```python
from build123d import *

# Parameters (mm, degrees)
F2_R      = 4
F2_R_2    = 3.4
F5_DEPTH  = 14
F7_R      = 15
F3_R      = 4
F4_R      = 3.2
F8_R      = 14.2
F6_R      = 15
F6_R_2    = 14.4
F11_DEPTH = 44
F14_DEPTH = 2.4
F15_R     = 15
F16_DEPTH = 0.6


with BuildPart() as f5:
    # F2 (on Top) → F5 (new body)
    with BuildSketch(Plane.XY):
        Circle(F2_R)
        Circle(F2_R_2, mode=Mode.SUBTRACT)
    extrude(amount=F5_DEPTH)

    # F7 (on offset) → F9 section 0
    with BuildSketch(Plane.XY.offset(-10)):
        Circle(F7_R)
    # F3 (on Top) → F9 section 1
    with BuildSketch(Plane.XY):
        Circle(F3_R)
    loft()

    # F4 (on Top) → F10 section 0
    with BuildSketch(Plane.XY):
        Circle(F4_R)
    # F8 (on offset) → F10 section 1
    with BuildSketch(Plane.XY.offset(-10)):
        Circle(F8_R)
    loft(mode=Mode.SUBTRACT)

    # F6 (on offset) → F11 (join)
    with BuildSketch(Plane.XY.offset(-10)):
        Circle(F6_R)
        Circle(F6_R_2, mode=Mode.SUBTRACT)
    extrude(amount=-F11_DEPTH)

    # F13 (on offset) → F14 (join)
    with BuildSketch(Plane(origin=(0, 0, -54), x_dir=(1, 0, 0), z_dir=(0, 0, -1))):
        with BuildLine():
            Line((0.3464101615, 0), (7.7583074711, 12.8377827207))
            ThreePointArc((7.7583074711, 12.8377827207), (7.5, 12.9903810568), (7.2386922288, 13.1377827207))
            Line((7.2386922288, 13.1377827207), (-0.1732050808, 0.3))
            Line((-0.1732050808, 0.3), (-14.9969996999, 0.3))
            ThreePointArc((-14.9969996999, 0.3), (-15, 0), (-14.9969996999, -0.3))
            Line((-14.9969996999, -0.3), (-0.1732050808, -0.3))
            Line((-0.1732050808, -0.3), (7.2386922288, -13.1377827207))
            ThreePointArc((7.2386922288, -13.1377827207), (7.5, -12.9903810568), (7.7583074711, -12.8377827207))
            Line((7.7583074711, -12.8377827207), (0.3464101615, 0))
        make_face()
    extrude(amount=-F14_DEPTH)

    # F15 (on offset) → F16 (join)
    with BuildSketch(Plane(origin=(0, 0, -54), x_dir=(1, 0, 0), z_dir=(0, 0, -1))):
        Circle(F15_R)
    extrude(amount=F16_DEPTH)


solid = f5.part
```
The model under review builds one solid part; all positions refer to its coordinate system, in mm. A direction names the side the tool comes from. Give positions to 0.01 mm unless a question says otherwise; leave off trailing zeros. Write each loop counter-clockwise with the first axis right and the second up, starting at its lowest first coordinate (ties: lowest second). Pieces come first, ordered by that corner, then holes. Notation, with made-up numbers: M 78.5,35.25 L 110.5,35.25 A20 cw 110.5,53.25 Z; hole C -31,10.5 d8. An arc over 180 degrees is marked long. Write item = value, one per line. Start each with the question number.
Q1. For line 1 (X direction, y = 0, z = -33.5); line 2 (Y direction, x = 0, z = 7.75), list the stretches that pass through material, from the lowest coordinate up.
Q2. We need section A-A (z = -5.5). State the section outline as (x, y) points.
Q3. Clearance check with flat-ended pins moving along their axes: pin 1 (0.7 mm diameter, centred on x = -7, z = -53, fed in from -Y); pin 2 (1.5 mm diameter, centred on x = 9.5, z = -37, fed in from +Y); pin 3 (4 mm diameter, centred on x = 11.5, y = 1, fed in from +Z). State where each tip first meets the part, or that it passes through.
Q4. Machinability: for faces 1 (the face through (-0.74, -3.32, 6.9)), 2 (the face through (-2, -3, 14)), 3 (the face through (-4, -7, -54)), which of the approach directions +Z, -Z, +X, -X, +Y, -Y give a long, thin tool a straight path to every point of the face, cutting with its end or side? Answer none if there is none.
Q5. We need section B-B (z = -37). State the section outline as (x, y) points, plus the area to 3 significant figures.
Q6. Mouldability with a two-part tool opening along X and no side actions: class faces 4 (the face through (-0.59, 4.5, -0.49)), 5 (the face through (3.432, -6.545, -52.817)), 6 (the face through (0, 0, -54.6)) as released by +X, released by -X, zero draft, split by the parting line, or undercut.
Result set:
q1.line_1 = -15 to -14.4, 14.4 to 15
q1.line_2 = -4 to -3.4, 3.4 to 4
q2.outline = C 0,0 d20.1; hole C 0,0 d18.5
q3.pin_1 = -13.45
q3.pin_2 = 12.18
q3.pin_3 = -5.04
q4.face_1 = +Z
q4.face_2 = +Z, +X, -X, +Y, -Y
q4.face_3 = none
q5.outline = C 0,0 d30; hole C 0,0 d28.8
q5.area = 55.4 mm2
q6.face_4 = split by the parting line
q6.face_5 = undercut
q6.face_6 = zero draft
